For this review, use the dimensioned drawing (mm, ordinates from the lowest corner) and the shaded views. A direction names the side the tool comes from. Give positions to 0.01 mm unless a question says otherwise; leave off trailing zeros. Loops run counter-clockwise (first coordinate to the right, second up) from the corner with the lowest first, then second, coordinate; pieces in that order, holes last. Notation, with made-up numbers: M 26.25,-9.5 L 58.25,-9.5 A28 ccw 58.25,10.5 Z; hole C -16.75,53 d11. An arc over 180 degrees is marked long. Use a Markdown table: item, result. Add a question column.
(1) Draft analysis for pull direction X (two halves, no side actions). For the marked faces 3, 4 and 5, state which applies: pulls with the +X half, pulls with the -X half, needs draft (parallel to the pull), parting line crosses it, or undercut.
(2) Add section A-A, the plane y = 44.45. Give the boundary of the cut face in (x, z) (1 decimal), then the cut area to 3 significant figures.
(3) For probe 1 along X at (y, z) = (44, 31); probe 2 along X at (y, z) = (48.5, 42) (1 decimal); probe 3 along X at (y, z) = (55, 23), list the stretches that pass through material, from the lowest coordinate up.
(4) Insertion check: pin 1 Ø12 at (x, z) = (18, 40.5) entering from +Y; pin 2 Ø1.5 at (y, z) = (22, 27.5) entering from +X; pin 3 Ø6 at (y, z) = (61.5, 31) entering from -X; pin 4 Ø1 at (y, z) = (57, 18.5) entering from +X (1 decimal). Each pin has a flat end and moves straight along its axis. Give the tip position at first contact, or say it passes through.
(5) For the marked faces 1 and 2, list the 3-axis set-ups (+Z, -Z, +X, -X, +Y, -Y) from which the entire face can be reached by the end or side of a thin tool; tool diameter is ignored.
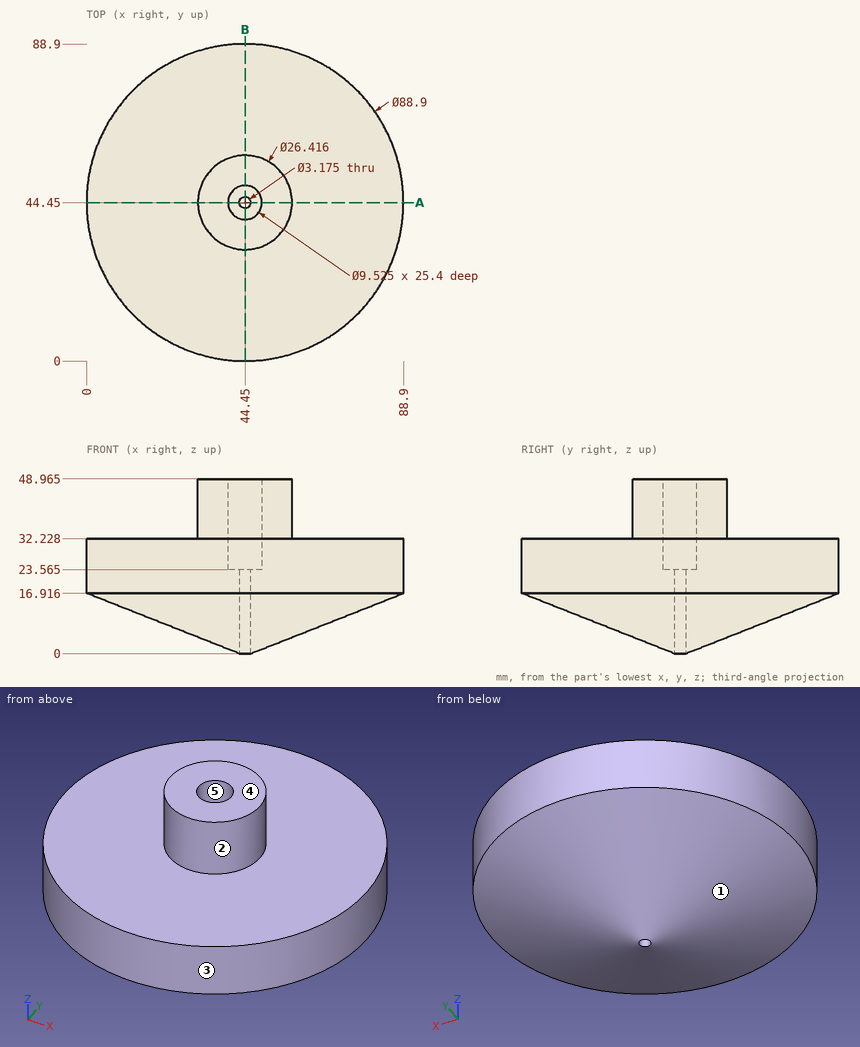
Established:
| question | item | result |
|---|---|---|
| 1 | face 3 | parting line crosses it |
| 1 | face 4 | needs draft |
| 1 | face 5 | undercut |
| 2 | outline | M 0,16.9 L 42.9,0 L 42.9,23.6 L 39.7,23.6 L 39.7,49 L 31.2,49 L 31.2,32.2 L 0,32.2 Z; M 46,0 L 88.9,16.9 L 88.9,32.2 L 57.7,32.2 L 57.7,49 L 49.2,49 L 49.2,23.6 L 46,23.6 Z |
| 2 | area | 2,270 mm^2 |
| 3 | probe 1 | 0 to 39.71, 49.19 to 88.9 |
| 3 | probe 2 | 31.9 to 41.9, 47 to 57 |
| 3 | probe 3 | 1.27 to 87.63 |
| 4 | pin 1 | through |
| 4 | pin 2 | x = 83.24 |
| 4 | pin 3 | x = 2.28 |
| 4 | pin 4 | x = 87.2 |
| 5 | face 1 | -Z |
| 5 | face 2 | +Z |
